```python
from build123d import *

# Parameters (mm, degrees)
ESQUISSE1_W             = 40
ESQUISSE1_H             = 20
ESQUISSE1_R             = 4
BOSS_EXTRU_1_DEPTH      = 50
ESQUISSE2_W             = 12
ESQUISSE2_H             = 5
ENL_V_MAT_EXTRU_1_DEPTH = 5
ESQUISSE3_R             = 1.5
ENL_V_MAT_EXTRU_2_DEPTH = 8
CONG_2_R                = 6
CONG_3_R                = 2


with BuildPart() as part:
    # Esquisse1 → Boss.-Extru.1 (new body)
    with BuildSketch(Plane.XY):
        Rectangle(ESQUISSE1_W, ESQUISSE1_H)
        with Locations((-10, 0)):
            Circle(ESQUISSE1_R, mode=Mode.SUBTRACT)
        with Locations((10, 0)):
            Circle(ESQUISSE1_R, mode=Mode.SUBTRACT)
    extrude(amount=BOSS_EXTRU_1_DEPTH)

    # Esquisse2 → Enlèv. mat.-Extru.1 (cut)
    with BuildSketch(Plane.XY.offset(50)):
        with Locations((-14, -7.5)):
            Rectangle(ESQUISSE2_W, ESQUISSE2_H)
        with Locations((14, -7.5)):
            Rectangle(ESQUISSE2_W, ESQUISSE2_H)
    enl_v_mat_extru_1 = extrude(amount=-ENL_V_MAT_EXTRU_1_DEPTH, mode=Mode.SUBTRACT)

    # Esquisse3 → Enlèv. mat.-Extru.2 (cut)
    with BuildSketch(Plane.XY.offset(45)):
        with Locations((-17, -7.5)):
            Circle(ESQUISSE3_R)
        with Locations(Location((-11, -7.5, 0), (0, 0, 180))):
            Circle(ESQUISSE3_R)
        with Locations(Location((17, -7.5, 0), (0, 0, 180))):
            Circle(ESQUISSE3_R)
        with Locations((11, -7.5)):
            Circle(ESQUISSE3_R)
    enl_v_mat_extru_2 = extrude(amount=-ENL_V_MAT_EXTRU_2_DEPTH, mode=Mode.SUBTRACT)

    # Symétrie1: Enlèv. mat.-Extru.1, Enlèv. mat.-Extru.2 across plane
    add(enl_v_mat_extru_1.mirror(Plane.XY.offset(25)), mode=Mode.SUBTRACT)
    add(enl_v_mat_extru_2.mirror(Plane.XY.offset(25)), mode=Mode.SUBTRACT)

    # Congé2
    cong_2_edges = [part.edges().sort_by_distance(p)[0] for p in [
        (-20, 10, 25),
        (20, 10, 25),
    ]]
    fillet(cong_2_edges, radius=CONG_2_R)

    # Congé3
    cong_3_edges = [part.edges().sort_by_distance(p)[0] for p in [
        (20, -10, 25),
        (-20, -10, 25),
    ]]
    fillet(cong_3_edges, radius=CONG_3_R)


solid = part.part
```
Verification items for the finished model (mm, model axes). A direction names the side the tool comes from. Coordinates: 2 decimals unless noted, no trailing zeros. Order: outer loops, then holes, each group sorted by start corner. A loop starts at its lowest first (then second) coordinate and runs counter-clockwise, first axis right, second up. Notation, with made-up numbers: (4, 1) -> (34, 1) arc R23 ccw to (34, 29) -> close; hole circle Ø9 at (62, -32). An arc over 180 degrees is marked (long way). Put each result on its own line as item: value. Start each with the question number.
1) Tool access check on faces 1 (the flat face through (14, -7, 45)), 2 (the cylindrical face through (18.2, -6.6, 8.9)), 3 (the flat face through (-14, -7, 45)). Record the directions out of +Z, -Z, +X, -X, +Y, -Y that give a thin tool (end or side, any length) a straight path to the whole face; none if there is none.
2) Release check for a two-part mould opening along X. For faces 4 (the flat face through (-17, -7, 37)), 5 (the flat face through (-8, -8, 2)), 6 (the flat face through (-14, -7, 5)) record: pulls with the +X half, pulls with the -X half, needs draft (parallel to the pull), parting line crosses it, or undercut.
3) Cross-section at B-B (y = 0). Enter the section's corners in (x, z), plus the area to 3 significant figures.
4) Cross-section at C-C (x = 11). Enter the section's corners in (y, z), plus the area to 3 significant figures.
5) Cross-section at A-A (z = 36). Enter the section's corners in (x, y).
6) Material ranges on L1, parallel to Y at x = 11, z = 41.25; L2, parallel to Y at x = 10, z = 11; L3, parallel to Y at x = -10, z = 28.5, recorded low to high.
7) Go/stop test with flat-tipped pins: pin 1 (1.5 mm diameter, centred on x = 12.5, y = -6.5, fed in from +Z); pin 2 (0.9 mm diameter, centred on x = 17.5, y = -7.5, fed in from -Z); pin 3 (2.5 mm diameter, centred on x = 11, y = -7, fed in from -Z); pin 4 (5 mm diameter, centred on x = -10, y = 0, fed in from +Z). Record where each tip stops, or that it passes through.
8) Cross-section at D-D (x = -17). Enter the section's corners in (y, z), plus the area to 3 significant figures.
Geometry check:
1. face 1: +Z, +X, -Y
1. face 2: -Z
1. face 3: +Z, -X, -Y
2. face 4: undercut
2. face 5: pulls with the -X half
2. face 6: needs draft
3. outline: (-20, 0) -> (-14, 0) -> (-14, 50) -> (-20, 50) -> close; (-6, 0) -> (6, 0) -> (6, 50) -> (-6, 50) -> close; (14, 0) -> (20, 0) -> (20, 50) -> (14, 50) -> close
3. area: 1,200 mm^2
4. outline: (-10, 5) -> (-9, 5) -> (-9, 13) -> (-6, 13) -> (-6, 5) -> (-5, 5) -> (-5, 0) -> (-3.87, 0) -> (-3.87, 50) -> (-5, 50) -> (-5, 45) -> (-6, 45) -> (-6, 37) -> (-9, 37) -> (-9, 45) -> (-10, 45) -> close; (3.87, 0) -> (10, 0) -> (10, 50) -> (3.87, 50) -> close
4. area: 515 mm^2
5. outline: (-20, -8) arc R2 ccw to (-18, -10) -> (18, -10) arc R2 ccw to (20, -8) -> (20, 4) arc R6 ccw to (14, 10) -> (-14, 10) arc R6 ccw to (-20, 4) -> close; hole circle Ø8 at (-10, 0); hole circle Ø8 at (10, 0)
6. L1: y = -10 to -9, -6 to -3.87, 3.87 to 10
6. L2: y = -10 to -8.62, -6.38 to -4, 4 to 10
6. L3: y = -10 to -4, 4 to 10
7. pin 1: stops at z = 45
7. pin 2: stops at z = 13
7. pin 3: stops at z = 5
7. pin 4: passes through
8. outline: (-10, 5) -> (-9, 5) -> (-9, 13) -> (-6, 13) -> (-6, 5) -> (-5, 5) -> (-5, 0) -> (9.2, 0) -> (9.2, 50) -> (-5, 50) -> (-5, 45) -> (-6, 45) -> (-6, 37) -> (-9, 37) -> (-9, 45) -> (-10, 45) -> close
8. area: 862 mm^2
